from build123d import *

# Parameters (mm, degrees)
F0_W     = 76.2
F0_H     = 863.6
F1_DEPTH = 9.525
F2_W     = 12.7
F2_H     = 69.85
F3_DEPTH = 38.1
F2_H_2   = 44.45
F4_DEPTH = 38.1
F5_DEPTH = 38.1
F6_W     = 12.7
F6_H     = 19.05
F7_DEPTH = 25.4


with BuildPart() as f1:
    # F0 (on Front) → F1 (new body, symmetric)
    with BuildSketch(Plane.XZ):
        Rectangle(F0_W, F0_H)
    extrude(amount=F1_DEPTH, both=True)

    # F2 (on face) → F3 (cut)
    with BuildSketch(Plane.YZ.offset(38.1)):
        with Locations((0, 393.7)):
            Rectangle(F2_W, F2_H)
    extrude(amount=-F3_DEPTH, mode=Mode.SUBTRACT)

    # F2 (on face) → F4 (cut)
    with BuildSketch(Plane.YZ.offset(38.1)):
        Rectangle(F2_W, F2_H_2)
    extrude(amount=-F4_DEPTH, mode=Mode.SUBTRACT)

    # F2 (on face) → F5 (cut)
    with BuildSketch(Plane.YZ.offset(38.1)):
        with Locations((0, -393.7)):
            Rectangle(F2_W, F2_H)
    extrude(amount=-F5_DEPTH, mode=Mode.SUBTRACT)

    # F6 (on face) → F7 (cut)
    with BuildSketch(Plane.YZ.offset(38.1)):
        with Locations((0, 190.5)):
            Rectangle(F6_W, F6_H)
    extrude(amount=-F7_DEPTH, mode=Mode.SUBTRACT)


solid = f1.part
Geometry: final body of the model. Coordinates: model frame, mm. A direction names the side the tool comes from. Round coordinates to 2 decimals unless told otherwise and drop trailing zeros. Loops run counter-clockwise (first coordinate to the right, second up) from the corner with the lowest first, then second, coordinate; pieces in that order, holes last. Notation, with made-up numbers: M -15,-30.75 L -10,-30.75 A32 cw -10,-0.75 Z; hole C -28,22.5 d6. An arc over 180 degrees is marked long. One line per question, with ' | ' between items.
(1) Cut plane B-B on y = -1.75. Return the cut outline in (x, z) (3 decimals).
Check result:
outline: M -38.1,-431.8 L 38.1,-431.8 L 38.1,-428.625 L 0,-428.625 L 0,-358.775 L 38.1,-358.775 L 38.1,-22.225 L 0,-22.225 L 0,22.225 L 38.1,22.225 L 38.1,180.975 L 12.7,180.975 L 12.7,200.025 L 38.1,200.025 L 38.1,358.775 L 0,358.775 L 0,428.625 L 38.1,428.625 L 38.1,431.8 L -38.1,431.8 Z
(2) Pull-direction query (Z, two-part tool) for faces 3 (the flat face through (19, 6.35, -394)), 4 (the flat face through (-1, 0, -431.8)), 5 (the flat face through (-1, 9.525, 6)); classes: +Z half, -Z half, draft (parallel to the pull), parting line (faces both ways), or undercut.
Check result:
face 3: undercut | face 4: -Z half | face 5: draft
(3) Material intervals for line 1 along Z through (x, y) = (4, -2.5) (3 decimals); line 2 along Z through (x, y) = (25.5, -3.5) (3 decimals); line 3 along Y through (x, z) = (30.5, -387) (3 decimals), sorted ascending. Write a range as from..to.
Check result:
line 1: z = -431.8..-428.625, -358.775..-22.225, 22.225..358.775, 428.625..431.8 | line 2: z = -431.8..-428.625, -358.775..-22.225, 22.225..180.975, 200.025..358.775, 428.625..431.8 | line 3: y = -9.525..-6.35, 6.35..9.525
(4) Access query for faces 1 (the flat face through (-38.1, 0, -6)), 2 (the flat face through (19, 6.35, 0)). Directions: +Z, -Z, +X, -X, +Y, -Y. A direction counts if a zero-diameter tool reaches every point of the face in a straight line with its end or side. Return the directions, or none.
Check result:
face 1: +Z, -Z, -X, +Y, -Y | face 2: +X
(5) Cut plane A-A on x = 21.5. Return the cut outline in (y, z) (3 decimals), plus the area to 3 significant figures.
Check result:
outline: M -9.525,-431.8 L 9.525,-431.8 L 9.525,431.8 L -9.525,431.8 Z; hole M -6.35,-428.625 L 6.35,-428.625 L 6.35,-358.775 L -6.35,-358.775 Z; hole M -6.35,-22.225 L 6.35,-22.225 L 6.35,22.225 L -6.35,22.225 Z; hole M -6.35,180.975 L 6.35,180.975 L 6.35,200.025 L -6.35,200.025 Z; hole M -6.35,358.775 L 6.35,358.775 L 6.35,428.625 L -6.35,428.625 Z | area: 13,900 mm2
(6) Contact query for flat-ended pins moving along their axis: P1, Ø10, axis at y = -0.5, z = 192.5, coming from the +X side; P2, Ø4, axis at y = -1, z = -389, coming from the +X side. Output: stop coordinate, or through.
Check result:
P1: stops at x = 12.7 | P2: stops at x = 0
